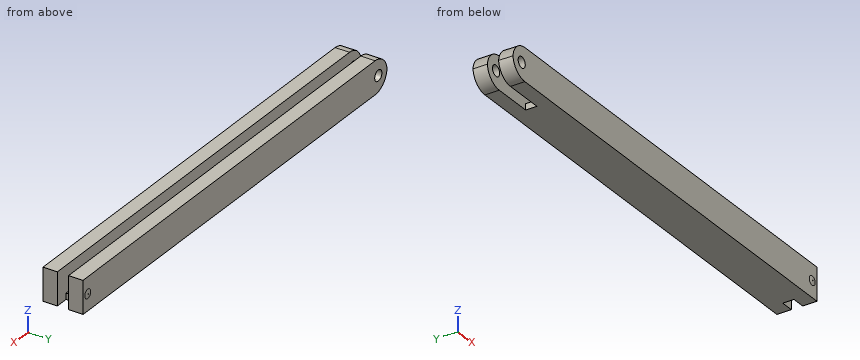
from build123d import *

# Parameters (mm, degrees)
F0_W        = 129.5146
F0_H        = 11.303
F1_DEPTH    = 9.271
F2_W        = 206.3660303733
F2_H        = 3.175
F3_DEPTH    = 7.5438
F4_W        = 3.7084
F4_H        = 3.175
F5_DEPTH    = 25.4
F6_W        = 16.3322
F6_H        = 3.175
F7_DEPTH    = 25.4
F8_T1_DEPTH = 29.464
F8_T3_DEPTH = 29.464
F9_R        = 1.524
F10_DEPTH   = 25.4
F12_DEPTH   = 0.127


# Not quite as in the source:
# - a fillet or chamfer that OpenCascade refuses, or shapes differently, is made with other operations: its cross-section is extruded or revolved along the edge and cut away or added


with BuildPart() as f1:
    # F0 (on Top) → F1 (new body)
    with BuildSketch(Plane.XY):
        Rectangle(F0_W, F0_H)
    extrude(amount=F1_DEPTH)

    # F2 (on face) → F3 (cut)
    with BuildSketch(Plane.XY.offset(9.271)):
        Rectangle(F2_W, F2_H)
    extrude(amount=-F3_DEPTH, mode=Mode.SUBTRACT)

    # F4 (on face) → F5 (cut)
    with BuildSketch(Plane.XY.offset(1.7272)):
        with Locations((62.9031, 0)):
            Rectangle(F4_W, F4_H)
    extrude(amount=-F5_DEPTH, mode=Mode.SUBTRACT)

    # F6 (on face) → F7 (cut)
    with BuildSketch(Plane.XY.offset(1.7272)):
        with Locations((-56.5912, 0)):
            Rectangle(F6_W, F6_H)
    extrude(amount=-F7_DEPTH, mode=Mode.SUBTRACT)

    # F8: fillet of radius 5.08 on 4 edges, made by hand

    # F8_s2 → F8_t1 (cut)
    with BuildSketch(Plane.XZ.offset(-11.1125)):
        with BuildLine():
            ThreePointArc((-64.7573, 4.191), (-63.2694024484, 7.7831024484), (-59.6773, 9.271))
            Line((-59.6773, 9.271), (-64.7573, 9.271))
            Line((-64.7573, 9.271), (-64.7573, 4.191))
        make_face()
        with BuildLine():
            ThreePointArc((-64.7573, 5.08), (-63.2694024484, 1.4878975516), (-59.6773, 0))
            Line((-59.6773, 0), (-64.7573, 0))
            Line((-64.7573, 0), (-64.7573, 5.08))
        make_face()
    extrude(amount=F8_T1_DEPTH, mode=Mode.SUBTRACT)

    # F8_s4 → F8_t3 (cut)
    with BuildSketch(Plane.XZ.offset(-18.3515)):
        with BuildLine():
            ThreePointArc((-59.6773, 9.271), (-63.2694024484, 7.7831024484), (-64.7573, 4.191))
            Line((-64.7573, 4.191), (-64.7573, 9.271))
            Line((-64.7573, 9.271), (-59.6773, 9.271))
        make_face()
        with BuildLine():
            ThreePointArc((-64.7573, 5.08), (-63.2694024484, 1.4878975516), (-59.6773, 0))
            Line((-59.6773, 0), (-64.7573, 0))
            Line((-64.7573, 0), (-64.7573, 5.08))
        make_face()
    extrude(amount=F8_T3_DEPTH, mode=Mode.SUBTRACT)

    # F9 (on face) → F10 (cut)
    with BuildSketch(Plane.XZ.offset(5.6515)):
        with Locations((-61.0294157593, 4.6167229302)):
            Circle(F9_R)
    extrude(amount=-F10_DEPTH, mode=Mode.SUBTRACT)

    # F11 (on face) → F12 (join)
    with BuildSketch(Plane.XZ.offset(5.6515)):
        with BuildLine():
            Line((61.4553, 4.6355), (63.9953, 4.6355))
            ThreePointArc((63.9953, 4.6355), (62.7253, 5.9055), (61.4553, 4.6355))
        make_face()
        with BuildLine():
            ThreePointArc((61.4553, 4.6355), (62.7253, 3.3655), (63.9953, 4.6355))
            Line((63.9953, 4.6355), (61.4553, 4.6355))
        make_face()
    extrude(amount=F12_DEPTH)

    # F13: fillet of radius 5.08 on 1 edges, made by hand

    # F13_s1 → F13_t2 (revolve, cut)
    with BuildSketch(Plane.XY.offset(4.6355)):
        with BuildLine():
            ThreePointArc((61.4553, -5.6515), (62.0161394247, -5.7466501562), (62.584100691, -5.7785))
            Line((62.584100691, -5.7785), (61.4553, -5.7785))
            Line((61.4553, -5.7785), (61.4553, -5.6515))
        make_face()
    revolve(axis=Axis((62.7253, -5.7785, 4.6355), (0, -1, 0)), mode=Mode.SUBTRACT)

    # F14: F1 across plane


with BuildPart() as f1_1:
    add(f1.part)
    add(f1.part.mirror(Plane.XZ))


solid = f1_1.part
For this review, take the finished solid that the model builds, in its own axes (mm). Round coordinates to 2 decimals unless told otherwise and drop trailing zeros. Loops run counter-clockwise (first coordinate to the right, second up) from the corner with the lowest first, then second, coordinate; pieces in that order, holes last. Notation, with made-up numbers: (-31.5, 63.5) - (-14.5, 63.5) arc R23 ccw to (-14.5, 102.5) - close; hole circle Ø9 at (40, 64.5). An arc over 180 degrees is marked (long way). Use one line per item in the form item = value.
1) Clearance check with flat-ended pins moving along their axes: P1, Ø2.5, axis at x = -8.5, y = 0, coming from the +Z side; P2, Ø2, axis at x = 18.5, z = 5, coming from the -Y side; P3, Ø1.5, axis at y = -3, z = 1.5, coming from the -X side. State where each tip first meets the part, or that it passes through.
Solutions:
P1 = 1.73
P2 = -5.65
P3 = -63.9
2) Wall thickness on probe 1 along Y at (x, z) = (32.5, 8); probe 2 along Y at (x, z) = (15, 1); probe 3 along Z at (x, y) = (-36, 0.5): over which ranges is each line inside the solid? List them lowest first.
Solutions:
probe_1 = -5.65 to -1.59, 1.59 to 5.65
probe_2 = -5.65 to 5.65
probe_3 = 0 to 1.73
3) We need section B-B on y = 0.5. Write out the cut boundary in (x, z).
Solutions:
outline = (-48.43, 0) - (61.05, 0) - (61.05, 1.73) - (-48.43, 1.73) - close
4) We need section A-A on x = 51. Write out the cut boundary in (y, z), then the cut area to 3 significant figures.
Solutions:
outline = (-5.65, 0) - (5.65, 0) - (5.65, 9.27) - (1.59, 9.27) - (1.59, 1.73) - (-1.59, 1.73) - (-1.59, 9.27) - (-5.65, 9.27) - close
area = 80.8 mm2
